Design review of the part built by this model. Coordinates are the model's own, in mm. A direction names the side the tool comes from. Coordinates: 2 decimals unless noted, no trailing zeros. Loops run counter-clockwise (first coordinate to the right, second up) from the corner with the lowest first, then second, coordinate; pieces in that order, holes last. Notation, with made-up numbers: (61.25, 21.5) - (104.25, 21.5) arc R21 cw to (104.25, 36.5) - close; hole circle Ø7 at (28.5, 85.5). An arc over 180 degrees is marked (long way). Answer in a Markdown table with one row per item. Add a question column.
(1) We need section B-B, the plane y = -28. Write out the cut boundary in (x, z).
(2) We need section D-D, the plane z = 29. Write out the cut boundary in (x, y).
(3) Clearance check with flat-ended pins moving along their axes: pin 1 (6.5 mm diameter, centred on x = -3.5, y = -17, fed in from -Z); pin 2 (2 mm diameter, centred on y = -1, z = 5, fed in from -X); pin 3 (2 mm diameter, centred on x = 1, z = 7, fed in from -Y); pin 4 (1.8 mm diameter, centred on x = 0, y = -16, fed in from +Z). State where each tip first meets the part, or that it passes through.
(4) For faces 4 (the face through (-2.03, -25.93, 41.67)), 5 (the face through (-0.028, -7.262, 27.147)), 6 (the face through (-8.014, -8.363, 32.419)), 7 (the face through (0.2, -17.3, 40)), list the 3-axis set-ups (+Z, -Z, +X, -X, +Y, -Y) from which the entire face can be reached by the end or side of a thin tool; tool diameter is ignored.
(5) We need section A-A, the plane z = 10.5. Write out the cut boundary in (x, y), plus the area to 3 significant figures.
(6) We need section C-C, the plane y = -16. Write out the cut boundary in (x, z), plus the area to 3 significant figures.
(7) The part is to be moulded in two halves that separate along X. For faces 1 (the face through (2, -26.02, 41.62)), 2 (the face through (-0.028, -3.054, -3.462)), 3 (the face through (-6.001, -13.228, 41.622)), say which applies: released by +X, released by -X, zero draft, split by the parting line, or undercut.
(8) To check wall thickness, follow L1, parallel to Y at x = 0, z = 39.4; L2, parallel to Z at x = -10, y = -20; L3, parallel to Y at x = -8.25, z = 8. State the ranges of each line that lie inside material, in increasing order. Write a range as [from, to].
Autodesk Inventor part; units mm, degrees
ref_plane "XZ Plane" through (0, 0, 0) normal (0, 1, 0) x (-1, 0, 0)
ref_plane "XY Plane" through (0, 0, 0) normal (0, 0, 1) x (1, 0, 0)
sketch "Sketch1" plane through (0, 0, 0) normal (0, 1, 0) x (-1, 0, 0)
  line L0 (-9, 40) -> (9, 40)
  line L1 (9, 40) -> (9, -9.6569)
  line L2 (9, -9.6569) -> (-9, -9.6569)
  line L3 (-9, -9.6569) -> (-9, 40)
  line L4 (-9, 40) -> (9, -9.6569) construction
  line L5 (9, 40) -> (-9, -9.6569) construction
  line L6 (0, -32.0453) -> (0, 52.0076) construction
  line L7 (-14.8076, 0) -> (25.8453, 0) construction
  line L8 (0, 0) -> (20.0378, -20.0378) construction
  line L9 (5.6569, -6.6569) -> (5.6569, 24.6569) construction
  line L10 (6.6569, -5.6569) -> (6.6569, 23.6569)
  line L11 (4.6569, 23.6569) -> (4.6569, -5.6569)
  arc A0 (4.6569, -5.6569) -> (6.6569, -5.6569) centre (5.6569, -5.6569) ccw
  arc A1 (6.6569, 23.6569) -> (4.6569, 23.6569) centre (5.6569, 23.6569) ccw
  line L12 (0, 0) -> (13.8345, 13.8345) construction
  line L13 (-5.6569, -6.6569) -> (-5.6569, 24.6569) construction
  line L14 (-6.6569, -5.6569) -> (-6.6569, 23.6569)
  line L15 (-4.6569, 23.6569) -> (-4.6569, -5.6569)
  arc A2 (-6.6569, -5.6569) -> (-4.6569, -5.6569) centre (-5.6569, -5.6569) ccw
  arc A3 (-4.6569, 23.6569) -> (-6.6569, 23.6569) centre (-5.6569, 23.6569) ccw
  point P0 (0, 15.1716)
  point P1 (0, 15.1716)
  point P2 (5.6569, -5.6569)
  point P3 (5.6569, 9)
  point P4 (5.6569, 5.6569)
  point P5 (-5.6569, -5.6569)
  point P6 (-5.6569, 9)
  point P7 (-5.6569, 5.6569)
  dimension "d34" = 18
  dimension "d35" = 45
  dimension "d36" = 8
  dimension "d37" = 2
  dimension "d38" = 0
  dimension "d40" = 45
  dimension "d41" = 18
  dimension "d42" = 4
  dimension "d43" = 40
extrude "Extrusion1" add sketch "Sketch1" against normal blind 2
sketch "Sketch4" plane through (-9, 0, 40) normal (0, 0, 1) x (1, 0, 0)
  line L0 (18, 0) -> (18, -2) construction
  line L1 (0, 0) -> (18, 0)
  line L2 (18, 0) -> (18, -17.6754)
  line L3 (9, -39.0627) -> (9, -2) construction
  line L4 (18, -2) -> (0, -2) construction
  line L5 (9, -24) -> (14.2107, -27.0084) construction
  circle A0 centre (15.9282, -28) radius 1
  circle A1 centre (9, -16) radius 1
  circle A2 centre (2.0718, -28) radius 1
  arc A3 (0, -17.6754) -> (18, -17.6754) centre (9, -24) ccw
  line L6 (0, -17.6754) -> (0, 0)
  point P0 (9, 0)
  dimension "d44" = 60
  dimension "d45" = 2
  dimension "d46" = 8
  dimension "d49" = 360
  dimension "d51" = 22
  dimension "d53" = 22
extrude "Extrusion4" add sketch "Sketch4" against normal blind 2
sketch "Sketch5" plane through (-9, -2, -9.6569) normal (-1, 0, 0) x (0, 0, 1)
  line L0 (47.6569, 0) -> (47.6569, -15.6754)
  line L1 (47.6569, -12.5494) -> (36.3362, 0)
  line L2 (47.6569, 0) -> (0, 0)
  line L3 (47.6569, 0) -> (47.6569, -12.5494)
  line L4 (47.6569, 0) -> (36.3362, 0)
  point P0 (9.6569, 2)
extrude "Extrusion5" add sketch "Sketch5" against normal blind 2
pattern_linear "Rectangular Pattern1" count 2 spacing 16 along (1, 0, 0) of "Extrusion5"
sketch "Sketch6" plane through (0, 0, 0) normal (1, 0, 0) x (0, 1, 0)
  line L0 (-14.5494, 38) -> (-2, 38) construction
  line L1 (-10.3568, 38) -> (-4.0789, 15.9865)
  line L2 (0, 40) -> (0, -9.6569)
  line L3 (-2, 38) -> (-10.3568, 38)
  line L4 (-4.0789, 15.9865) -> (-4.0789, -2.2693)
  line L5 (-4.0789, -2.2693) -> (-2, -4.6891)
  line L6 (-2, -4.6891) -> (-2, 38)
  point P0 (0, 0)
extrude "Extrusion6" add sketch "Sketch6" along normal mid plane 4
sketch "Sketch7" plane through (-9, 0, 40) normal (0, 0, 1) x (1, 0, 0)
  circle A0 centre (9, -16) radius 1 construction
  circle A1 centre (9, -16) radius 2 construction
  circle A2 centre (15.9282, -28) radius 1 construction
  circle A3 centre (15.9282, -28) radius 2 construction
  point P0 (9, 0)
  point P1 (14.689, -14.1786)
  point P2 (10.5252, -27.4837)
  dimension "d63" = 4
  dimension "d64" = 4
ref_plane "Work Plane2" through (1.5252, -27.4837, 40) normal (-0.9544, 0.2987, 0) x (0, 0, 1)
sketch "Sketch8" plane through (1.5252, -27.4837, 40) normal (-0.9544, 0.2987, 0) x (0, 0, 1)
  line L0 (0, 11.593) -> (0, -8.1309)
  line L1 (0, -1.506) -> (3.29, 4.6767)
  line L2 (3.29, 4.6767) -> (3.29, 10.9801)
  line L3 (3.29, 10.9801) -> (0, 18.7943)
  line L4 (0, 23.0857) -> (0, 6.217)
  line L5 (0, -1.506) -> (0, 18.7943)
  point P0 (-40, 25.7737)
extrude "Extrusion7" add sketch "Sketch8" along normal mid plane 2
mirror "Mirror1" about plane through (0, 0, 0) normal (1, 0, 0) of "Extrusion7"
properties part number "gimbal_yaw_brushless" material "ABS Plastic"
Responses:
| question | item | result |
|---|---|---|
| 1 | outline | (-10.25, 38) - (-7.93, 38) - (-7.93, 40) - (-10.25, 40) - close; (-5.93, 38) - (5.93, 38) - (5.93, 40) - (2.41, 40) - (2.41, 40.68) - (0.32, 40.35) - (0.32, 40) - (-0.32, 40) - (-0.32, 40.35) - (-2.41, 40.68) - (-2.41, 40) - (-5.93, 40) - close; (7.93, 38) - (10.25, 38) - (10.25, 40) - (7.93, 40) - close |
| 2 | outline | (-9, -4.57) - (-7, -4.57) - (-7, -2) - (-2, -2) - (-2, -7.79) - (2, -7.79) - (2, -2) - (7, -2) - (7, -4.57) - (9, -4.57) - (9, 0) - (-9, 0) - close |
| 3 | pin 1 | stops at z = 38 |
| 3 | pin 2 | stops at x = -9 |
| 3 | pin 3 | stops at y = -4.08 |
| 3 | pin 4 | passes through |
| 4 | face 4 | +Z, -Y |
| 4 | face 5 | -Z, -Y |
| 4 | face 6 | -Z, -X, -Y |
| 4 | face 7 | +Z |
| 5 | outline | (-9, -2) - (-6.66, -2) - (-6.66, 0) - (-9, 0) - close; (-4.66, -2) - (-2, -2) - (-2, -4.08) - (2, -4.08) - (2, -2) - (4.66, -2) - (4.66, 0) - (-4.66, 0) - close; (6.66, -2) - (9, -2) - (9, 0) - (6.66, 0) - close |
| 5 | area | 36.3 mm2 |
| 6 | outline | (-9, 38) - (-1, 38) - (-1, 40) - (-4.07, 40) - (-4.07, 42.98) - (-6.17, 42.71) - (-6.17, 40) - (-9, 40) - close; (1, 38) - (9, 38) - (9, 40) - (6.17, 40) - (6.17, 42.71) - (4.07, 42.98) - (4.07, 40) - (1, 40) - close |
| 6 | area | 43.9 mm2 |
| 7 | face 1 | undercut |
| 7 | face 2 | zero draft |
| 7 | face 3 | released by -X |
| 8 | L1 | y = [-35, -17], [-15, 0] |
| 8 | L2 | z = [38, 40] |
| 8 | L3 | y = [-2, 0] |
